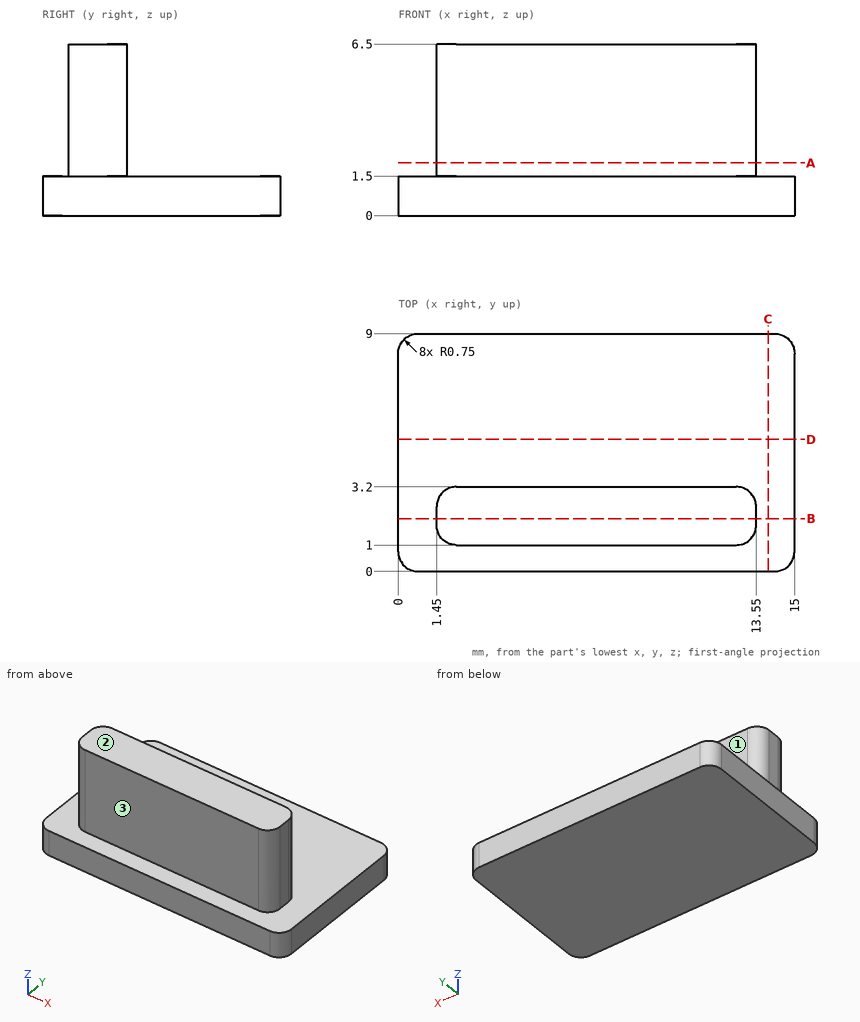
Could you check a few things on this drawing? It's one solid part, dimensions in mm from its lowest x, y, z. A direction names the side the tool comes from. Give positions to 0.01 mm unless a question says otherwise; leave off trailing zeros. Order: outer loops, then holes, each group sorted by start corner. A loop starts at its lowest first (then second) coordinate and runs counter-clockwise, first axis right, second up. Notation, with made-up numbers: (-9.5, -11.5) -> (21.5, -11.5) arc R22 ccw to (21.5, 20.5) -> close; hole circle Ø8 at (-23, 69.25). An arc over 180 degrees is marked (long way). Answer in a Markdown table with one row per item. Add a question column.
Item 1: For the marked faces 1, 2 and 3, which set-ups out of +Z, -Z, +X, -X, +Y, -Y let a thin tool reach every point of the face, with its end or its side?
Item 2: I'm going to push flat-ended pins straight in: P1, Ø0.6, axis at y = 2, z = 3, coming from the +X side; P2, Ø3, axis at x = 3.5, y = 7, coming from the -Z side; P3, Ø1, axis at x = 7, z = 5, coming from the +Y side. Where does each tip first touch, or does it pass through?
Item 3: Imagine slicing it at B-B (y = 2). List the corners of the cut face in (x, z) for me.
Item 4: Imagine slicing it at A-A (z = 2). List the corners of the cut face in (x, y) for me.
Item 5: Imagine slicing it at D-D (y = 5). List the corners of the cut face in (x, z) for me, and give its area (3 significant figures).
Item 6: Imagine slicing it at C-C (x = 14). List the corners of the cut face in (y, z) for me.
Item 7: Please list where these lines run through material, in increasing order: probe 1 along Y at (x, z) = (5.5, 4.75); probe 2 along Z at (x, y) = (2.5, 3.75); probe 3 along X at (y, z) = (1.25, 2.75).
Result:
| question | item | result |
|---|---|---|
| 1 | face 1 | +Z, +X, -X, +Y |
| 1 | face 2 | +Z, +X, -X, +Y, -Y |
| 1 | face 3 | +Z, +X, -X, -Y |
| 2 | P1 | x = 13.55 |
| 2 | P2 | z = 0 |
| 2 | P3 | y = 3.2 |
| 3 | outline | (0, 0) -> (15, 0) -> (15, 1.5) -> (13.55, 1.5) -> (13.55, 6.5) -> (1.45, 6.5) -> (1.45, 1.5) -> (0, 1.5) -> close |
| 4 | outline | (1.45, 1.75) arc R0.75 ccw to (2.2, 1) -> (12.8, 1) arc R0.75 ccw to (13.55, 1.75) -> (13.55, 2.45) arc R0.75 ccw to (12.8, 3.2) -> (2.2, 3.2) arc R0.75 ccw to (1.45, 2.45) -> close |
| 5 | outline | (0, 0) -> (15, 0) -> (15, 1.5) -> (0, 1.5) -> close |
| 5 | area | 22.5 mm2 |
| 6 | outline | (0, 0) -> (9, 0) -> (9, 1.5) -> (0, 1.5) -> close |
| 7 | probe 1 | 1 to 3.2 |
| 7 | probe 2 | 0 to 1.5 |
| 7 | probe 3 | 1.64 to 13.36 |
